from build123d import *

# Parameters (mm, degrees)
SKETCH_1_W                  = 20.04
SKETCH_1_H                  = 9.94
EXTRUDE_1_DEPTH             = 6.12
SKETCH_2_R                  = 0.25
EXTRUDE_2_DEPTH             = 4
PATTERN_LINEAR_1_COUNT      = 8
PATTERN_LINEAR_1_PITCH      = 2.54
PATTERN_LINEAR_1_COUNT_DIR2 = 2
PATTERN_LINEAR_1_PITCH_DIR2 = 7.62
SKETCH_3_W                  = 19.05
SKETCH_3_H                  = 8.89
CUT_EXTRUDE_1_DEPTH         = 0.01


with BuildPart() as part:
    # Эскиз1 → Бобышка-Вытянуть1 (new body)
    with BuildSketch(Plane.XY):
        Rectangle(SKETCH_1_W, SKETCH_1_H)
    extrude(amount=EXTRUDE_1_DEPTH)

    # Эскиз2 → Бобышка-Вытянуть2 (add)
    with BuildSketch(Plane(origin=(0, 0, 0), x_dir=(-1, 0, 0), z_dir=(0, 0, -1))):
        with Locations((8.89, -3.81)):
            Circle(SKETCH_2_R)
    extrude_2 = extrude(amount=EXTRUDE_2_DEPTH)

    # Линейный массив1: Extrude 2 8 × 2
    with Locations(*[(i * PATTERN_LINEAR_1_PITCH, j * PATTERN_LINEAR_1_PITCH_DIR2, 0) for i in range(PATTERN_LINEAR_1_COUNT) for j in range(PATTERN_LINEAR_1_COUNT_DIR2) if (i, j) != (0, 0)]):
        add(extrude_2)

    # Эскиз3 → Вырез-Вытянуть1 (cut)
    with BuildSketch(Plane.XY.offset(6.12)):
        Rectangle(SKETCH_3_W, SKETCH_3_H)
    extrude(amount=-CUT_EXTRUDE_1_DEPTH, mode=Mode.SUBTRACT)


solid = part.part
Read the model definition and answer for the solid it produces. Units are mm, in the model's axes. Round coordinates to 2 decimals unless told otherwise and drop trailing zeros. Loops run counter-clockwise (first coordinate to the right, second up) from the corner with the lowest first, then second, coordinate; pieces in that order, holes last. Notation, with made-up numbers: (-7, -40) - (1, -40) arc R15 cw to (1, -18) - close; hole circle Ø5 at (-29.5, 9). An arc over 180 degrees is marked (long way). One line per question, with ' | ' between items. Start each with the question number.
Q1. Section A-A on z = -1 is taken. Count the separate pieces of the cut face and the enclosed holes in it, plus the area to 3 significant figures.
Q2. Flat-ended cylindrical pins translate along their axes: pin 1 (2.5 mm diameter, centred on x = -1.5, y = -1, fed in from +Z); pin 2 (3 mm diameter, centred on x = -7.5, y = 1, fed in from -Z). Find the tip coordinate at first contact, or state that the pin passes through.
Q3. Section B-B on x = 1.27 is taken. Give the vertices of the cut face in (y, z) (3 decimals).
Q4. Section C-C on y = 1 is taken. Give the vertices of the cut face in (x, z) (3 decimals).
Q5. Find the intervals of material crossed by L1, parallel to Z at x = 2, y = -0.25, in increasing order.
Established:
1) separate pieces: 16 | enclosed holes: 0 | area: 3.14 mm²
2) pin 1: z = 6.11 | pin 2: z = 0
3) outline: (-4.97, 0) - (-4.06, 0) - (-4.06, -4) - (-3.56, -4) - (-3.56, 0) - (3.56, 0) - (3.56, -4) - (4.06, -4) - (4.06, 0) - (4.97, 0) - (4.97, 6.12) - (4.445, 6.12) - (4.445, 6.11) - (-4.445, 6.11) - (-4.445, 6.12) - (-4.97, 6.12) - close
4) outline: (-10.02, 0) - (10.02, 0) - (10.02, 6.12) - (9.525, 6.12) - (9.525, 6.11) - (-9.525, 6.11) - (-9.525, 6.12) - (-10.02, 6.12) - close
5) L1: 0 to 6.11
